The listing builds one solid part. Answer for the finished solid, in the listing's coordinates (mm). Face numbers are marked on the shaded views. A direction names the side the tool comes from. Coordinates: 2 decimals unless noted, no trailing zeros. Order: outer loops, then holes, each group sorted by start corner. A loop starts at its lowest first (then second) coordinate and runs counter-clockwise, first axis right, second up. Notation, with made-up numbers: (-15.75, 34.25) -> (10.25, 34.25) arc R7 cw to (10.25, 38.25) -> close; hole circle Ø9 at (-33, 82.25). An arc over 180 degrees is marked (long way). Answer in a Markdown table with one row per item. Add a question column.
```python
from build123d import *

# Parameters (mm, degrees)
F0_R     = 38.1
F0_R_2   = 25.4
F1_DEPTH = 50.8
F2_W     = 67.6658935845
F2_H     = 55.8053161949
F3_DEPTH = 12.7
F5_DEPTH = 38.1
F7_DEPTH = 25.4


with BuildPart() as f1:
    # F0 (on Top) → F1 (new body)
    with BuildSketch(Plane.XY):
        with Locations((38.0283864189, 0)):
            Circle(F0_R)
        with Locations((38.0283864189, 0)):
            Circle(F0_R_2, mode=Mode.SUBTRACT)
    extrude(amount=F1_DEPTH)

    # F2 (on Top) → F3 (join)
    with BuildSketch(Plane.XY):
        with Locations((-21.5929765254, 0.0276817009)):
            Rectangle(F2_W, F2_H)
    extrude(amount=F3_DEPTH)

    # F4 (on face) → F5 (join)
    with BuildSketch(Plane.XY.offset(12.7)):
        with BuildLine():
            ThreePointArc((0.0846197344, -3.4468202446), (-0.0698650899, 0.3650095571), (0.1576249962, 4.1731797554))
            Line((0.1576249962, 4.1731797554), (-40.3746258327, 4.1731797554))
            Line((-40.3746258327, 4.1731797554), (-40.3746258327, -3.4468202446))
            Line((-40.3746258327, -3.4468202446), (0.0846197344, -3.4468202446))
        make_face()
    extrude(amount=F5_DEPTH)

    # F6 (on face) → F7 (cut)
    with BuildSketch(Plane.XZ.offset(3.4468202446)):
        Polygon((-40.3746258327, 12.7), (0.0846197344, 50.8), (-40.3746258327, 50.8), align=None)
    extrude(amount=-F7_DEPTH, mode=Mode.SUBTRACT)


solid = f1.part
```
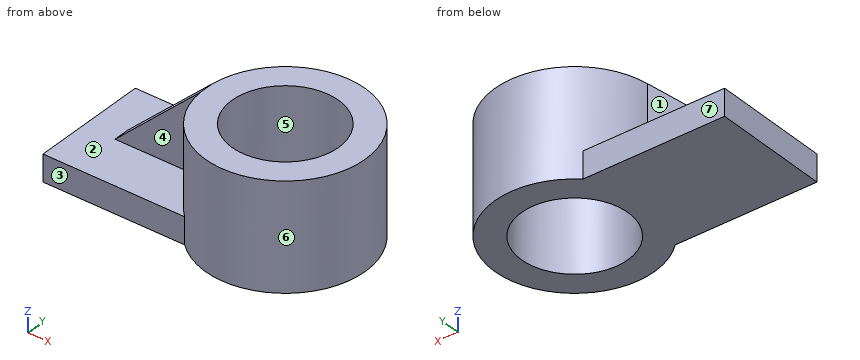
Q1. A cutting plane is placed at C-C (x = -9.5). Determine the outline of the cut face in (y, z).
Q2. Given pin 1 (3 mm diameter, centred on x = -11, y = -15.5, fed in from +Z); pin 2 (4 mm diameter, centred on y = -28, z = 27.5, fed in from -X); pin 3 (10 mm diameter, centred on x = -37, z = 3.5, fed in from +Y), each flat-ended and moving along its own axis, determine where each tip first touches the part or whether it passes through.
Q3. Straight lines are drawn through the part: line 1 (Z direction, x = -33, y = -5.5); line 2 (X direction, y = -13, z = 10); line 3 (X direction, y = 13, z = 13.5). For each, find the intervals that lie inside material, in ascending order.
Q4. A cutting plane is placed at B-B (z = 7.5). Determine the outline of the cut face in (x, y).
Q5. A cutting plane is placed at D-D (y = -15.5). Determine the outline of the cut face in (x, z).
Q6. For the marked faces 1, 2 and 3, determine the directions among +Z, -Z, +X, -X, +Y, -Y from which every point of the face is accessible in a straight line to the end or side of a thin tool.
Q7. Determine the mould class of the marked faces 4, 5, 6 and 7 for opening direction Y: +Y half, -Y half, draft (parallel to the pull), parting line (faces both ways), or undercut.
Q8. A cutting plane is placed at A-A (y = 0). Determine the outline of the cut face in (x, z), then the cut area to 3 significant figures.
Returned:
| question | item | result |
|---|---|---|
| 1 | outline | (-27.87, 0) -> (27.93, 0) -> (27.93, 12.7) -> (4.17, 12.7) -> (4.17, 41.77) -> (-3.45, 41.77) -> (-3.45, 12.7) -> (-27.87, 12.7) -> close |
| 2 | pin 1 | stops at z = 12.7 |
| 2 | pin 2 | stops at x = 10.18 |
| 2 | pin 3 | stops at y = 27.93 |
| 3 | line 1 | z = 0 to 12.7 |
| 3 | line 2 | x = -55.43 to 16.21, 59.85 to 73.84 |
| 3 | line 3 | x = 2.21 to 16.21, 59.85 to 73.84 |
| 4 | outline | (-55.43, -27.87) -> (12.06, -27.87) arc R38.1 ccw (long way) to (12.11, 27.93) -> (-55.43, 27.93) -> close; hole circle Ø50.8 at (38.03, 0) |
| 5 | outline | (-55.43, 0) -> (17.91, 0) -> (17.91, 50.8) -> (3.22, 50.8) -> (3.22, 12.7) -> (-55.43, 12.7) -> close; (58.15, 0) -> (72.83, 0) -> (72.83, 50.8) -> (58.15, 50.8) -> close |
| 6 | face 1 | +Z, -X, +Y |
| 6 | face 2 | +Z, -X |
| 6 | face 3 | +Z, -Z, -X, -Y |
| 7 | face 4 | -Y half |
| 7 | face 5 | undercut |
| 7 | face 6 | parting line |
| 7 | face 7 | +Y half |
| 8 | outline | (-55.43, 0) -> (12.63, 0) -> (12.63, 50.8) -> (0.08, 50.8) -> (-40.37, 12.7) -> (-55.43, 12.7) -> close; (63.43, 0) -> (76.13, 0) -> (76.13, 50.8) -> (63.43, 50.8) -> close |
| 8 | area | 2,760 mm² |
